```python
from build123d import *

# Parameters (mm, degrees)
F0_R     = 12
F1_DEPTH = 10
F2_DEPTH = 5
F3_R     = 12
F3_W     = 5.38
F3_H     = 5.38
F4_DEPTH = 20


with BuildPart() as f1:
    # F0 (on Right) → F1 (new body)
    with BuildSketch(Plane.YZ):
        Circle(F0_R)
        Polygon((0, 7.147596), (6.19, 3.573798), (6.19, -3.573798), (0, -7.147596), (-6.19, -3.573798), (-6.19, 3.573798), align=None, mode=Mode.SUBTRACT)
    extrude(amount=F1_DEPTH)

    # F0 (on Right) → F2 (join)
    with BuildSketch(Plane.YZ):
        Circle(F0_R)
        Polygon((0, 7.147596), (6.19, 3.573798), (6.19, -3.573798), (0, -7.147596), (-6.19, -3.573798), (-6.19, 3.573798), align=None, mode=Mode.SUBTRACT)
        Polygon((6.19, -3.573798), (6.19, 3.573798), (0, 7.147596), (-6.19, 3.573798), (-6.19, -3.573798), (0, -7.147596), align=None)
    extrude(amount=-F2_DEPTH)

    # F3 (on face) → F4 (join)
    with BuildSketch(Plane(origin=(-5, 0, 0), x_dir=(0, -1, 0), z_dir=(-1, 0, 0))):
        Circle(F3_R)
        Rectangle(F3_W, F3_H, mode=Mode.SUBTRACT)
    extrude(amount=F4_DEPTH)


solid = f1.part
```
Input: part model. Units: mm. Frame: model coordinates. A direction names the side the tool comes from. Coordinates: 2 decimals unless noted, no trailing zeros. Order: outer loops, then holes, each group sorted by start corner. A loop starts at its lowest first (then second) coordinate and runs counter-clockwise, first axis right, second up. Notation, with made-up numbers: (48.5, -28.5) - (62.5, -28.5) arc R13 cw to (62.5, -10.5) - close; hole circle Ø11 at (13.25, 59.5). An arc over 180 degrees is marked (long way). Put each result on its own line as item: value.
1. Cut plane A-A on z = 0. Return the cut outline in (x, y).
Report:
outline: (-25, -12) - (10, -12) - (10, -6.19) - (0, -6.19) - (0, 6.19) - (10, 6.19) - (10, 12) - (-25, 12) - (-25, 2.69) - (-5, 2.69) - (-5, -2.69) - (-25, -2.69) - close
2. Cut plane B-B on x = -11.5. Return the cut outline in (y, z), then the cut area to 3 significant figures.
Report:
outline: circle Ø24 at (0, 0); hole (-2.69, -2.69) - (2.69, -2.69) - (2.69, 2.69) - (-2.69, 2.69) - close
area: 423 mm2
3. Line query: line 1 along X through (y, z) = (2.75, -2.75); line 2 along Y through (x, z) = (2, 0); line 3 along Z through (x, y) = (2, 3.75). Output: solid intervals per line, ascending.
Report:
line 1: x = -25 to 0
line 2: y = -12 to -6.19, 6.19 to 12
line 3: z = -11.4 to -4.98, 4.98 to 11.4
4. Contact query for flat-ended pins moving along their axis: pin 1 Ø5 at (x, z) = (-3.5, -5) entering from -Y; pin 2 Ø2.5 at (y, z) = (-1, 1) entering from -X; pin 3 Ø1 at (x, y) = (-7, -6) entering from -Z. Output: stop coordinate, or through.
Report:
pin 1: stops at y = -11.74
pin 2: stops at x = -5
pin 3: stops at z = -10.67
5. Draft query along Z for faces 1 (the face through (-15, 0, -2.69)), 2 (the face through (10, 5, -5)). Return one class per face: pulls with the +Z half, pulls with the -Z half, needs draft (parallel to the pull), parting line crosses it, or undercut.
Report:
face 1: undercut
face 2: needs draft
6. Cut plane D-D on y = -10.25. Return the cut outline in (x, z), then the cut area to 3 significant figures.
Report:
outline: (-25, -6.24) - (10, -6.24) - (10, 6.24) - (-25, 6.24) - close
area: 437 mm2
7. Cut plane C-C on y = -5. Return the cut outline in (x, z), then the cut area to 3 significant figures.
Report:
outline: (-25, -10.91) - (10, -10.91) - (10, -4.26) - (0, -4.26) - (0, 4.26) - (10, 4.26) - (10, 10.91) - (-25, 10.91) - close
area: 678 mm2
8. Reachability of faces 3 (the face through (-25, 0, 3)), 4 (the face through (-15, -2.69, 0)), 5 (the face through (4.93, 3.052, 5.386)) from +Z, -Z, +X, -X, +Y, -Y: full face, straight path, thin tool, end or side. Return the list, or none.
Report:
face 3: +Z, -Z, -X, +Y, -Y
face 4: -X
face 5: +X
